Design review of the part built by this model. Coordinates are the model's own, in mm. Round coordinates to 2 decimals unless told otherwise and drop trailing zeros. Loops run counter-clockwise (first coordinate to the right, second up) from the corner with the lowest first, then second, coordinate; pieces in that order, holes last. Notation, with made-up numbers: (8, -3) -> (63, -3) arc R18 ccw to (63, 27) -> close; hole circle Ø3 at (-15.75, 53). An arc over 180 degrees is marked (long way). Write each question's results on one line, items separated by ' | '. Start each with the question number.
from build123d import *

# Parameters (mm, degrees)
SKETCH_1_R      = 1.5
EXTRUDE_1_DEPTH = 3
CHAMFER_1_SIZE  = 1.5


with BuildPart() as part:
    # 草图1 → 凸台-拉伸1 (new body)
    with BuildSketch(Plane(origin=(0, 0, 0), x_dir=(1, 0, 0), z_dir=(0, 1, 0))):
        with BuildLine():
            Line((-48.265241636, 51.265241636), (-48.265241636, -51.265241636))
            ThreePointArc((-48.265241636, -51.265241636), (-50.117191339, -54.036880234), (-53.38656198, -53.38656198))
            ThreePointArc((-53.38656198, -53.38656198), (-75.5, 0), (-53.38656198, 53.38656198))
            ThreePointArc((-53.38656198, 53.38656198), (-50.117191339, 54.036880234), (-48.265241636, 51.265241636))
        make_face()
        with Locations(Location((-51.265241636, -51.265241636, 0), (0, 0, 270))):
            Circle(SKETCH_1_R, mode=Mode.SUBTRACT)
        with Locations(Location((-72.5, 0, 0), (0, 0, 270))):
            Circle(SKETCH_1_R, mode=Mode.SUBTRACT)
        with Locations(Location((-51.265241636, 51.265241636, 0), (0, 0, 270))):
            Circle(SKETCH_1_R, mode=Mode.SUBTRACT)
        with Locations(Location((-61.499999084, -25.5, 0), (0, 0, 270))):
            Circle(SKETCH_1_R, mode=Mode.SUBTRACT)
        with Locations(Location((-53.499999084, -25.5, 0), (0, 0, 270))):
            Circle(SKETCH_1_R, mode=Mode.SUBTRACT)
        with Locations(Location((-61.499999084, 25.5, 0), (0, 0, 270))):
            Circle(SKETCH_1_R, mode=Mode.SUBTRACT)
        with Locations(Location((-53.499999084, 25.5, 0), (0, 0, 270))):
            Circle(SKETCH_1_R, mode=Mode.SUBTRACT)
    extrude(amount=EXTRUDE_1_DEPTH)

    # 倒角1
    chamfer_1_edges = [part.edges().sort_by_distance(p)[0] for p in [
        (-72.5, 3, -1.5),
    ]]
    chamfer(chamfer_1_edges, length=CHAMFER_1_SIZE - 0.0001)  # a hair under: the kernel refuses the full size


solid = part.part
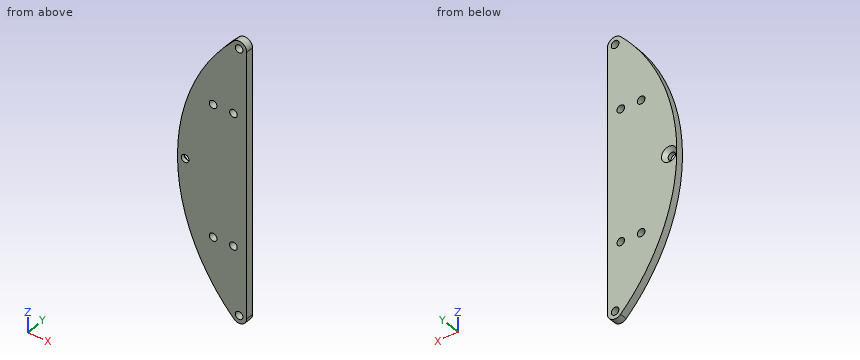
1) Take a section at D-D (x = -72.5). Write out the cut boundary in (y, z).
2) Insertion check: pin 1 (1 mm diameter, centred on x = -66, y = 1, fed in from +Z); pin 2 (1.5 mm diameter, centred on y = 2, z = 8.5, fed in from -X). Each pin has a flat end and moves straight along its axis. Give the tip position at first contact, or say it passes through.
3) Take a section at C-C (y = 2.3). Write out the cut boundary in (x, z), plus the area to 3 significant figures.
4) Take a section at B-B (x = -61.5). Write out the cut boundary in (y, z).
5) To check wall thickness, follow line 1 (Z direction, x = -61.25, y = 2.2); line 2 (X direction, y = 1.5, z = 25.5); line 3 (Z direction, x = -50.5, y = 0.8). State the ranges of each line that lie inside material, in increasing order. Write a range as from..to.
Geometry check:
1) outline: (0, -21.07) -> (3, -21.07) -> (3, -3) -> (1.5, -1.5) -> (0, -1.5) -> close; (0, 1.5) -> (1.5, 1.5) -> (3, 3) -> (3, 21.07) -> (0, 21.07) -> close
2) pin 1: stops at z = 37.55 | pin 2: stops at x = -75.1
3) outline: (-53.39, -53.39) arc R3 ccw to (-48.27, -51.27) -> (-48.27, 51.27) arc R3 ccw to (-53.39, 53.39) arc R75.5 ccw to start; hole circle Ø4.6 at (-72.5, 0); hole circle Ø3 at (-61.5, -25.5); hole circle Ø3 at (-61.5, 25.5); hole circle Ø3 at (-53.5, -25.5); hole circle Ø3 at (-53.5, 25.5); hole circle Ø3 at (-51.27, -51.27); hole circle Ø3 at (-51.27, 51.27) | area: 2,120 mm^2
4) outline: (0, -43.79) -> (3, -43.79) -> (3, -27) -> (0, -27) -> close; (0, -24) -> (3, -24) -> (3, 24) -> (0, 24) -> close; (0, 27) -> (3, 27) -> (3, 43.79) -> (0, 43.79) -> close
5) line 1: z = -44.14..-26.98, -24.02..24.02, 26.98..44.14 | line 2: x = -71.06..-63, -60..-55, -52..-48.27 | line 3: z = -54.17..-52.56, -49.98..49.98, 52.56..54.17
